```python
from build123d import *

# Parameters (mm, degrees)
SKETCH1_W           = 30
SKETCH1_H           = 30
SKETCH1_R           = 3.9
BOSS_EXTRUDE1_DEPTH = 3
SKETCH2_R           = 3.9
BOSS_EXTRUDE2_DEPTH = 3.2
SKETCH3_W           = 40
SKETCH3_H           = 40
BOSS_EXTRUDE3_DEPTH = 3


with BuildPart() as part:
    # Sketch1 → Boss-Extrude1 (new body)
    # profile 1 of 5: a face of its own
    with BuildSketch(Plane(origin=(0, 0, 0), x_dir=(1, 0, 0), z_dir=(0, 1, 0))):
        Rectangle(SKETCH1_W, SKETCH1_H)
        with Locations((10, -10)):
            Circle(SKETCH1_R, mode=Mode.SUBTRACT)
        with Locations((-10, -10)):
            Circle(SKETCH1_R, mode=Mode.SUBTRACT)
        with Locations((10, 10)):
            Circle(SKETCH1_R, mode=Mode.SUBTRACT)
        with Locations((-10, 10)):
            Circle(SKETCH1_R, mode=Mode.SUBTRACT)
    # profile 2 of 5: a face of its own
    with BuildSketch(Plane(origin=(0, 0, 0), x_dir=(1, 0, 0), z_dir=(0, 1, 0))):
        with Locations((-10, 10)):
            Circle(SKETCH1_R)
    # profile 3 of 5: a face of its own
    with BuildSketch(Plane(origin=(0, 0, 0), x_dir=(1, 0, 0), z_dir=(0, 1, 0))):
        with Locations((10, 10)):
            Circle(SKETCH1_R)
    # profile 4 of 5: a face of its own
    with BuildSketch(Plane(origin=(0, 0, 0), x_dir=(1, 0, 0), z_dir=(0, 1, 0))):
        with Locations((-10, -10)):
            Circle(SKETCH1_R)
    # profile 5 of 5: a face of its own
    with BuildSketch(Plane(origin=(0, 0, 0), x_dir=(1, 0, 0), z_dir=(0, 1, 0))):
        with Locations((10, -10)):
            Circle(SKETCH1_R)
    extrude(amount=BOSS_EXTRUDE1_DEPTH)

    # Sketch2 → Boss-Extrude2 (add)
    with BuildSketch(Plane(origin=(0, 3, 0), x_dir=(1, 0, 0), z_dir=(0, 1, 0))):
        with Locations(Location((-10, -10, 0), (0, 0, 270))):
            Circle(SKETCH2_R)
        with Locations(Location((10, -10, 0), (0, 0, 270))):
            Circle(SKETCH2_R)
        with Locations(Location((10, 10, 0), (0, 0, 270))):
            Circle(SKETCH2_R)
        with Locations(Location((-10, 10, 0), (0, 0, 270))):
            Circle(SKETCH2_R)
    extrude(amount=BOSS_EXTRUDE2_DEPTH)

    # Sketch3 → Boss-Extrude3 (add)
    with BuildSketch(Plane.XZ):
        Rectangle(SKETCH3_W, SKETCH3_H)
    extrude(amount=BOSS_EXTRUDE3_DEPTH)


solid = part.part
```
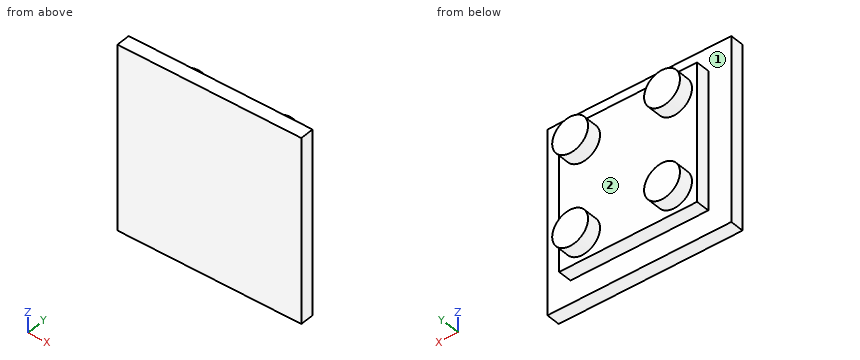
CAD build for the part. Positions are in the model's coordinates, mm. Face numbers are marked on the shaded views. Round coordinates to 2 decimals unless told otherwise and drop trailing zeros. Write each loop counter-clockwise with the first axis right and the second up, starting at its lowest first coordinate (ties: lowest second). Pieces come first, ordered by that corner, then holes. Notation, with made-up numbers: (-10.5, 60) -> (39.5, 60) arc R19 cw to (39.5, 64) -> close; hole circle Ø8 at (-36.5, 8.25). An arc over 180 degrees is marked (long way). Answer in a Markdown table with one row per item. Add a question column.
Item 1: Saw through at C-C, the plane y = 3.5. Write the cut outline in (x, z).
Item 2: Mould opens along X. For the marked faces 1 and 2 say: pulls with the +X half, pulls with the -X half, needs draft (parallel to the pull), parting line crosses it, or undercut.
Item 3: Saw through at B-B, the plane x = 10. Write the cut outline in (y, z), then the cut area to 3 significant figures.
Item 4: Saw through at D-D, the plane z = -10. Write the cut outline in (x, y), then the cut area to 3 significant figures.
Item 5: Saw through at A-A, the plane z = 5.5. Write the cut outline in (x, y).
Item 6: Drop flat-ended pins along their axis: pin 1 Ø0.9 at (x, y) = (-5.5, 1.5) entering from +Z; pin 2 Ø1.5 at (y, z) = (4.5, 10) entering from -X; pin 3 Ø2 at (x, y) = (2, 2.5) entering from -Z. Give the stop position or say it passes through.
Item 7: Drill centre lines: line 1 (Y direction, x = 14, z = 6); line 2 (Y direction, x = 15.5, z = 14); line 3 (X direction, y = 1, z = 7.5). Where is each one in solid material? Low to high. Write a range as from..to.
Findings below:
| question | item | result |
|---|---|---|
| 1 | outline | circle Ø7.8 at (-10, -10); circle Ø7.8 at (-10, 10); circle Ø7.8 at (10, -10); circle Ø7.8 at (10, 10) |
| 2 | face 1 | needs draft |
| 2 | face 2 | undercut |
| 3 | outline | (-3, -20) -> (0, -20) -> (0, -15) -> (3, -15) -> (3, -13.9) -> (6.2, -13.9) -> (6.2, -6.1) -> (3, -6.1) -> (3, 6.1) -> (6.2, 6.1) -> (6.2, 13.9) -> (3, 13.9) -> (3, 15) -> (0, 15) -> (0, 20) -> (-3, 20) -> close |
| 3 | area | 260 mm^2 |
| 4 | outline | (-20, -3) -> (20, -3) -> (20, 0) -> (15, 0) -> (15, 3) -> (13.9, 3) -> (13.9, 6.2) -> (6.1, 6.2) -> (6.1, 3) -> (-6.1, 3) -> (-6.1, 6.2) -> (-13.9, 6.2) -> (-13.9, 3) -> (-15, 3) -> (-15, 0) -> (-20, 0) -> close |
| 4 | area | 260 mm^2 |
| 5 | outline | (-20, -3) -> (20, -3) -> (20, 0) -> (15, 0) -> (15, 3) -> (-15, 3) -> (-15, 0) -> (-20, 0) -> close |
| 6 | pin 1 | stops at z = 15 |
| 6 | pin 2 | stops at x = -13.9 |
| 6 | pin 3 | stops at z = -15 |
| 7 | line 1 | y = -3..3 |
| 7 | line 2 | y = -3..0 |
| 7 | line 3 | x = -15..15 |
